Check sheet for the modelled part. Datum: model origin and axes. Units: mm. Round coordinates to 2 decimals unless told otherwise and drop trailing zeros. Write each loop counter-clockwise with the first axis right and the second up, starting at its lowest first coordinate (ties: lowest second). Pieces come first, ordered by that corner, then holes. Notation, with made-up numbers: (83.25, 19.5) -> (93.25, 19.5) arc R15 ccw to (93.25, 48.5) -> close; hole circle Ø5 at (45.5, -0.75). An arc over 180 degrees is marked (long way). One line per item, written item: value. Start each with the question number.
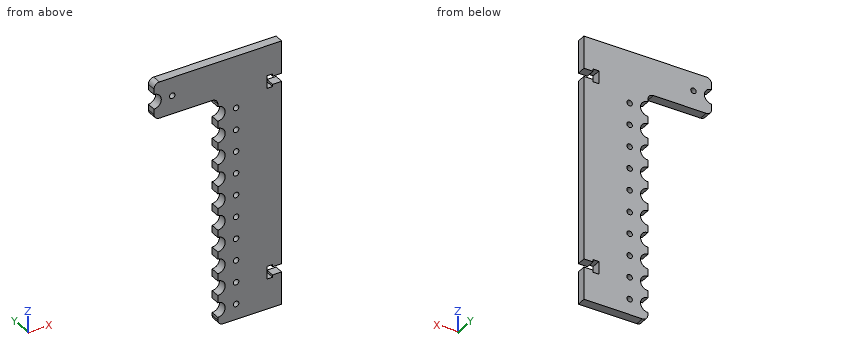
Autodesk Inventor part; units mm, degrees
ref_plane "YZ Plane" through (0, 0, 0) normal (1, 0, 0) x (0, 1, 0)
ref_plane "XZ Plane" through (0, 0, 0) normal (0, 1, 0) x (-1, 0, 0)
ref_plane "XY Plane" through (0, 0, 0) normal (0, 0, 1) x (1, 0, 0)
sketch "Sketch1" plane through (0, 0, 0) normal (0, 1, 0) x (-1, 0, 0)
  line L0 (0, 0) -> (70, 0)
  line L1 (70, 0) -> (70, -20)
  line L2 (70, -20) -> (35, -20)
  line L3 (35, -20) -> (35, -145)
  line L4 (35, -145) -> (0, -145)
  line L5 (0, -145) -> (0, 0)
  dimension "d0" = 35
  dimension "d1" = 145
  dimension "d2" = 70
  dimension "d3" = 20
extrude "Extrusion1" add sketch "Sketch1" along normal blind 5
sketch "Sketch2" plane through (0, 5, 0) normal (0, 1, 0) x (1, 0, 0)
  line L0 (-70, 20) -> (-70, 0)
  circle A0 centre (-70, 10) radius 4
  line L1 (-35, 145) -> (-35, 20)
  circle A1 centre (-35, 64.5) radius 4
  circle A2 centre (-35, 76.5) radius 4
  circle A3 centre (-35, 88.5) radius 4
  circle A4 centre (-35, 100.5) radius 4
  circle A5 centre (-35, 112.5) radius 4
  circle A6 centre (-35, 124.5) radius 4
  circle A7 centre (-35, 136.5) radius 4
  circle A8 centre (-35, 52.5) radius 4
  circle A9 centre (-35, 40.5) radius 4
  circle A10 centre (-35, 28.5) radius 4
  line L2 (0, 17.75) -> (0, 22.25)
  line L3 (0, 22.25) -> (-5, 22.25)
  line L4 (-5, 22.25) -> (-5, 23.5)
  line L5 (-5, 23.5) -> (-8.2, 23.5)
  line L6 (-8.2, 23.5) -> (-8.2, 16.5)
  line L7 (-8.2, 16.5) -> (-5, 16.5)
  line L8 (0, 17.75) -> (-5, 17.75)
  line L9 (-5, 17.75) -> (-5, 16.5)
  line L10 (0, 0) -> (0, 145)
  line L11 (0, 127.25) -> (-5, 127.25)
  line L12 (-5, 127.25) -> (-5, 128.5)
  line L13 (-5, 128.5) -> (-8.2, 128.5)
  line L14 (-8.2, 128.5) -> (-8.2, 121.5)
  line L15 (-8.2, 121.5) -> (-5, 121.5)
  line L16 (-5, 121.5) -> (-5, 122.75)
  line L17 (-5, 122.75) -> (0, 122.75)
  line L18 (0, 122.75) -> (0, 127.25)
  line L19 (-25, 28.5) -> (-25, 136.5) construction
  circle A11 centre (-25, 28.5) radius 1.5
  circle A12 centre (-25, 40.5) radius 1.5
  circle A13 centre (-25, 52.5) radius 1.5
  circle A14 centre (-25, 64.5) radius 1.5
  circle A15 centre (-25, 76.5) radius 1.5
  circle A16 centre (-25, 88.5) radius 1.5
  circle A17 centre (-25, 100.5) radius 1.5
  circle A18 centre (-25, 112.5) radius 1.5
  circle A19 centre (-25, 124.5) radius 1.5
  circle A20 centre (-25, 136.5) radius 1.5
  circle A21 centre (-60, 10) radius 1.5
  point P0 (-8.2, 125)
  point P1 (0, 125)
  point P2 (-8.2, 20)
  point P3 (0, 20)
  dimension "d6" = 8
  dimension "d7" = 8
  dimension "d8" = 8
  dimension "d9" = 8
  dimension "d11" = 8
  dimension "d12" = 8
  dimension "d13" = 8
  dimension "d14" = 8
  dimension "d15" = 8.5
  dimension "d16" = 12
  dimension "d17" = 12
  dimension "d18" = 12
  dimension "d19" = 12
  dimension "d20" = 12
  dimension "d21" = 12
  dimension "d22" = 8
  dimension "d23" = 8
  dimension "d24" = 12
  dimension "d25" = 12
  dimension "d26" = 12
  dimension "d27" = 8
  dimension "d28" = 7
  dimension "d29" = 3.2
  dimension "d30" = 4.5
  dimension "d31" = 5
  dimension "d32" = 3.2
  dimension "d33" = 5
  dimension "d34" = 7
  dimension "d35" = 4.5
  dimension "d36" = 20
  dimension "d37" = 20
  dimension "d38" = 3
  dimension "d39" = 3
  dimension "d40" = 3
  dimension "d41" = 3
  dimension "d42" = 3
  dimension "d43" = 3
  dimension "d44" = 3
  dimension "d45" = 3
  dimension "d46" = 3
  dimension "d47" = 3
  dimension "d48" = 10
  dimension "d52" = 3
  dimension "d53" = 10
extrude "Extrusion2" cut sketch "Sketch2" against normal blind 5
fillet "Fillet1" radius 3 4 edges at (-35, 2.5, -145) (-35, 2.5, -20) (-70, 2.5, -20) (-70, 2.5, 0)
properties part number "primary_holder" material "Polycarbonate, Clear"
1. Cross-section at B-B (x = -25). Give the number of separate pieces and of enclosed holes in the cut face, plus the area to 3 significant figures.
2. Material ranges on probe 1 along X at (y, z) = (3.5, -28.5); probe 2 along X at (y, z) = (2.9, -124.5); probe 3 along Z at (x, y) = (-60, 3.6), recorded low to high.
3. Depth check by flat-ended pin: pin 1 Ø5 at (x, z) = (-25, -100.5) entering from -Y; pin 2 Ø1.2 at (y, z) = (2.5, -57.5) entering from -X; pin 3 Ø3 at (y, z) = (3.5, -52.5) entering from -X; pin 4 Ø1 at (y, z) = (2.5, -101) entering from -X. Enter the tip coordinate at first touch or a pass-through.
4. Cross-section at C-C (z = -10). Record the cut outline in (x, y).
5. Cross-section at A-A (z = -124.5). Record the cut outline in (x, y), plus the area to 3 significant figures.
Working result:
1. separate pieces: 11
1. enclosed holes: 0
1. area: 575 mm^2
2. probe 1: x = -31 to -26.5, -23.5 to 0
2. probe 2: x = -31 to -26.5, -23.5 to -8.2
2. probe 3: z = -20 to -11.5, -8.5 to 0
3. pin 1: stops at y = 0
3. pin 2: stops at x = -35
3. pin 3: stops at x = -31.29
3. pin 4: stops at x = -31.13
4. outline: (-66, 0) -> (-61.5, 0) -> (-61.5, 5) -> (-66, 5) -> close; (-58.5, 0) -> (0, 0) -> (0, 5) -> (-58.5, 5) -> close
5. outline: (-31, 0) -> (-26.5, 0) -> (-26.5, 5) -> (-31, 5) -> close; (-23.5, 0) -> (-8.2, 0) -> (-8.2, 5) -> (-23.5, 5) -> close
5. area: 99.0 mm^2
